Autodesk Inventor part; units mm, degrees
ref_plane "Arbeitsebene3" through (-858.9244, 0, 0) normal (0, 0, 1) x (1, 0, 0)
ref_plane "YZ Plane" through (0, 0, 0) normal (1, 0, 0) x (0, 1, 0)
ref_plane "XZ Plane" through (0, 0, 0) normal (0, 1, 0) x (-1, 0, 0)
ref_plane "Arbeitsebene3" through (-858.9244, 0, 0) normal (0, 0, 1) x (1, 0, 0)
sketch "Skizze2" plane through (-858.9244, 0, 0) normal (0, 0, 1) x (1, 0, 0)
  line L0 (588.9244, 270) -> (1128.9244, 270)
  line L1 (1128.9244, 270) -> (1128.9244, -270)
  line L2 (1128.9244, -270) -> (588.9244, -270)
  line L3 (588.9244, -270) -> (588.9244, 270)
  line L4 (480.9244, 0) -> (1236.9244, 0)
  line L5 (858.9244, -378) -> (858.9244, 378)
  point P0 (858.9244, 0)
  dimension "d5" = 540
  dimension "d6" = 540
extrude "Extrusion2" add sketch "Skizze2" along normal blind 18
sketch "Skizze3" plane through (-858.9244, 0, 18) normal (0, 0, 1) x (1, 0, 0)
  line L0 (1128.9244, 270) -> (588.9244, 270)
  line L1 (588.9244, 270) -> (588.9244, -270)
  line L2 (588.9244, -270) -> (1128.9244, -270)
  line L3 (1128.9244, -270) -> (1128.9244, 270)
  line L4 (1110.9244, 252) -> (606.9244, 252)
  line L5 (606.9244, 252) -> (606.9244, -252)
  line L6 (606.9244, -252) -> (1110.9244, -252)
  line L7 (1110.9244, -252) -> (1110.9244, 252)
  point P0 (858.9244, 0)
  dimension "d12" = 18
  dimension "d13" = 18
  dimension "d14" = 18
  dimension "d15" = 18
extrude "Extrusion3" cut sketch "Skizze3" against normal blind 10
properties part number "Boden"
Geometry: final body of the model. Coordinates: model frame, mm. Round coordinates to 2 decimals unless told otherwise and drop trailing zeros. Loops run counter-clockwise (first coordinate to the right, second up) from the corner with the lowest first, then second, coordinate; pieces in that order, holes last. Notation, with made-up numbers: (68, -4.5) -> (107, -4.5) arc R13 cw to (107, 0.5) -> close; hole circle Ø7 at (75, -9). An arc over 180 degrees is marked (long way). Use one line per item in the form item = value.
Item 1: Cut plane C-C on z = 14. Output: boundary loops of the cut face in (x, y), then the cut area to 3 significant figures.
Evaluation:
outline = (-252, -252) -> (252, -252) -> (252, 252) -> (-252, 252) -> close
area = 254,000 mm2
Item 2: Contact query for flat-ended pins moving along their axis: pin 1 Ø8 at (y, z) = (46.5, 15) entering from +X; pin 2 Ø3 at (y, z) = (210, 16) entering from -X; pin 3 Ø5 at (x, z) = (80.5, 15) entering from +Y. Output: stop coordinate, or through.
Evaluation:
pin_1 = 252
pin_2 = -252
pin_3 = 252
Item 3: Material intervals for probe 1 along X at (y, z) = (55, 14.75), sorted ascending.
Evaluation:
probe_1 = -252 to 252
Item 4: Cut plane A-A on x = 1. Output: boundary loops of the cut face in (y, z).
Evaluation:
outline = (-270, 0) -> (270, 0) -> (270, 8) -> (252, 8) -> (252, 18) -> (-252, 18) -> (-252, 8) -> (-270, 8) -> close
